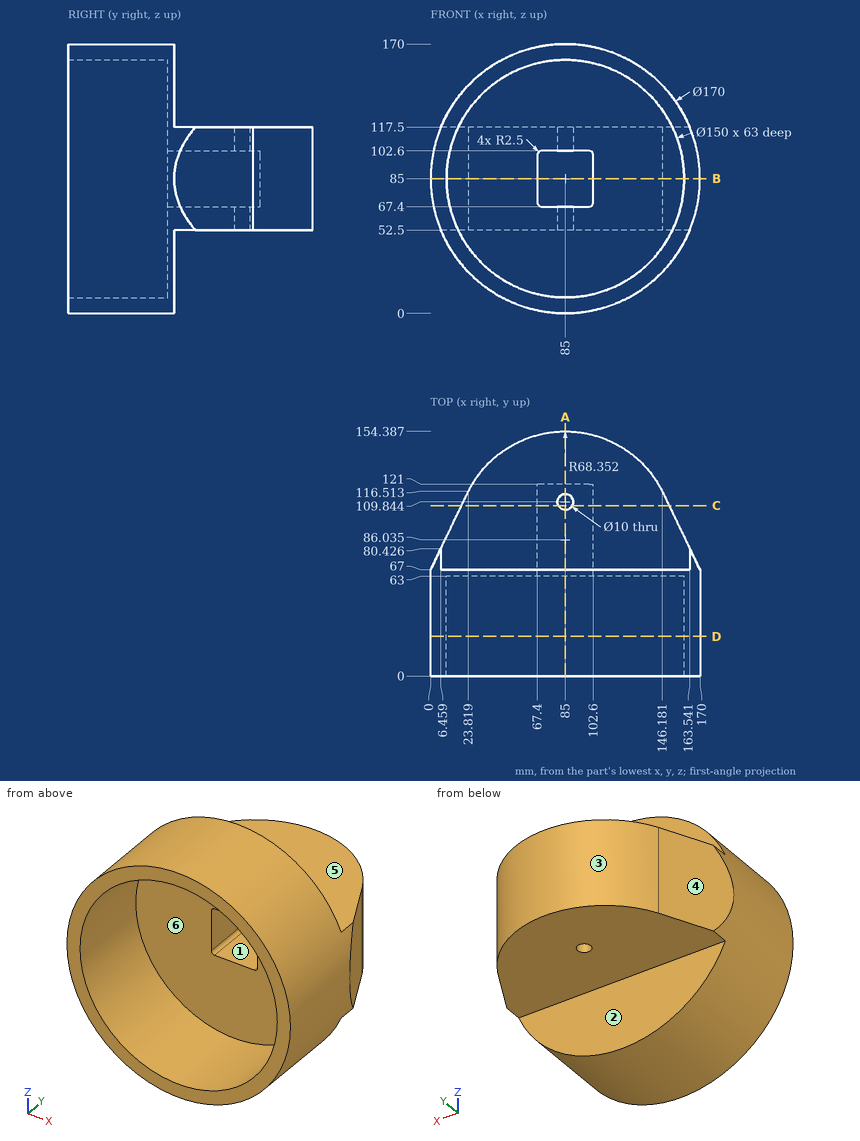
For this review, use the dimensioned drawing (mm, ordinates from the lowest corner) and the shaded views. A direction names the side the tool comes from. Round coordinates to 2 decimals unless told otherwise and drop trailing zeros. Write each loop counter-clockwise with the first axis right and the second up, starting at its lowest first coordinate (ties: lowest second). Pieces come first, ordered by that corner, then holes. Notation, with made-up numbers: (6.25, -16.5) -> (10.25, -16.5) arc R14 ccw to (10.25, 0.5) -> close; hole circle Ø10 at (10.25, -30). An arc over 180 degrees is marked (long way). One line per item, written item: value. Start each with the question number.
Q1. Tool access review of the marked faces 1, 2 and 3: name each direction out of +Z, -Z, +X, -X, +Y, -Y from which nothing blocks a thin tool from reaching the whole face with its end or side.
Q2. Insertion check: P1, Ø9, axis at x = 86, y = 90, coming from the -Z side; P2, Ø4, axis at x = 89, z = 88.5, coming from the -Y side; P3, Ø4, axis at y = 109.5, z = 96.5, coming from the -X side. Each pin has a flat end and moves straight along its axis. Give the tip position at first contact, or say it passes through.
Q3. Add section C-C (y = 107.5). Give the boundary of the cut face in (x, z), then the cut area to 3 significant figures.
Q4. Add section A-A (x = 85). Give the boundary of the cut face in (y, z) (1 decimal), then the cut area to 3 significant figures.
Q5. The part is to be moulded in two halves that separate along X. For the marked faces 4, 5 and 6, say which applies: pulls with the +X half, pulls with the -X half, needs draft (parallel to the pull), parting line crosses it, or undercut.
Q6. Add section D-D (y = 25). Give the boundary of the cut face in (x, z).
Q7. To check wall thickness, follow probe 1 along X at (y, z) = (30, 85); probe 2 along Y at (x, z) = (48, 157); probe 3 along Z at (x, y) = (129, 83.5). State the ranges of each line that lie inside material, in increasing order.
Q8. Add section B-B (z = 85). Give the boundary of the cut face in (x, y) (1 decimal).
Response:
1. face 1: -Y
1. face 2: -Z, +X, -X, +Y
1. face 3: +Z, -Z, +Y
2. P1: stops at z = 52.5
2. P2: stops at y = 121
2. P3: stops at x = 19.48
3. outline: (19.48, 52.5) -> (80.58, 52.5) -> (80.58, 67.4) -> (69.9, 67.4) arc R2.5 cw to (67.4, 69.9) -> (67.4, 100.1) arc R2.5 cw to (69.9, 102.6) -> (80.58, 102.6) -> (80.58, 117.5) -> (19.48, 117.5) -> close; (89.42, 52.5) -> (150.52, 52.5) -> (150.52, 117.5) -> (89.42, 117.5) -> (89.42, 102.6) -> (100.1, 102.6) arc R2.5 cw to (102.6, 100.1) -> (102.6, 69.9) arc R2.5 cw to (100.1, 67.4) -> (89.42, 67.4) -> close
3. area: 7,020 mm^2
4. outline: (0, 0) -> (67, 0) -> (67, 52.5) -> (104.8, 52.5) -> (104.8, 67.4) -> (63, 67.4) -> (63, 10) -> (0, 10) -> close; (0, 160) -> (63, 160) -> (63, 102.6) -> (104.8, 102.6) -> (104.8, 117.5) -> (67, 117.5) -> (67, 170) -> (0, 170) -> close; (114.8, 52.5) -> (154.4, 52.5) -> (154.4, 117.5) -> (114.8, 117.5) -> (114.8, 102.6) -> (121, 102.6) -> (121, 67.4) -> (114.8, 67.4) -> close
4. area: 5,280 mm^2
5. face 4: pulls with the -X half
5. face 5: needs draft
5. face 6: undercut
6. outline: circle Ø170 at (85, 85); hole circle Ø150 at (85, 85)
7. probe 1: x = 0 to 10, 160 to 170
7. probe 2: y = 0 to 67
7. probe 3: z = 52.5 to 117.5
8. outline: (0, 0) -> (10, 0) -> (10, 63) -> (67.4, 63) -> (67.4, 121) -> (102.6, 121) -> (102.6, 63) -> (160, 63) -> (160, 0) -> (170, 0) -> (170, 67) -> (146.2, 116.5) arc R68.4 ccw to (23.8, 116.5) -> (0, 67) -> close
